Geometry: see drawing. Coordinates: mm, zero at the bounding-box minimum. A direction names the side the tool comes from. Coordinates: 2 decimals unless noted, no trailing zeros. Order: outer loops, then holes, each group sorted by start corner. A loop starts at its lowest first (then second) coordinate and runs counter-clockwise, first axis right, second up.
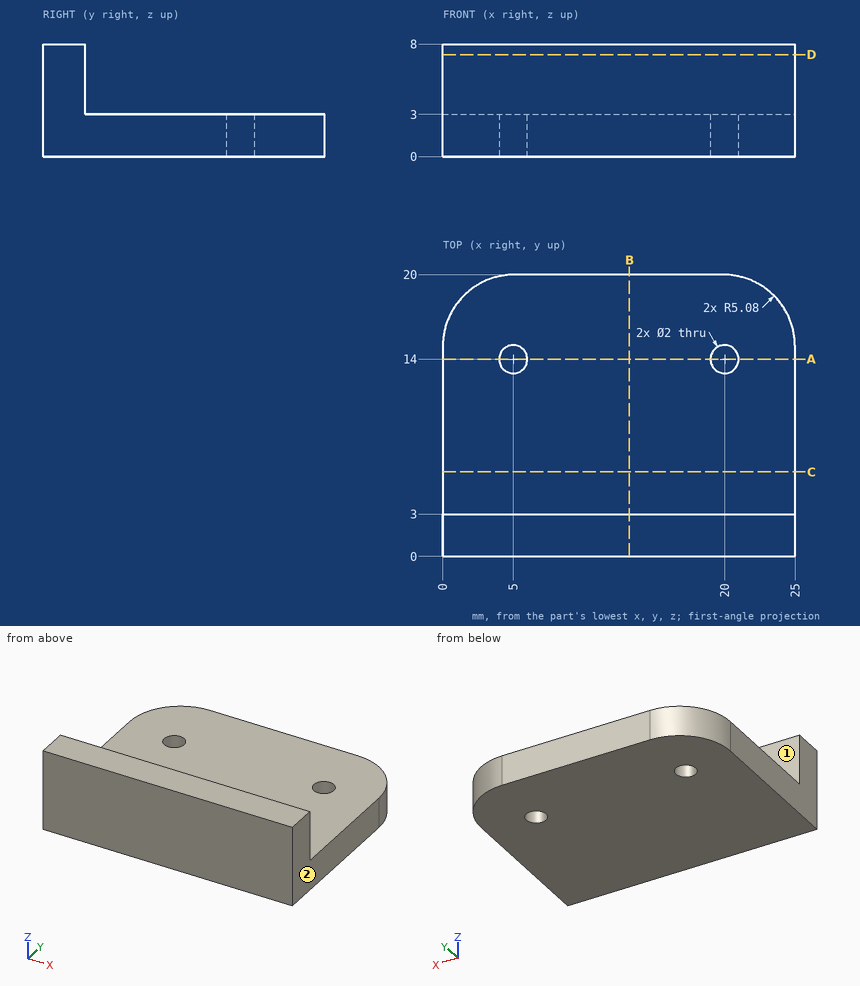
Item 1: Cut plane A-A on y = 14. Return loops of the section in (x, z).
Response values:
outline: (0, 0) - (4, 0) - (4, 3) - (0, 3) - close; (6, 0) - (19, 0) - (19, 3) - (6, 3) - close; (21, 0) - (25, 0) - (25, 3) - (21, 3) - close
Item 2: Cut plane C-C on y = 6. Return loops of the section in (x, z), then the cut area to 3 significant figures.
Response values:
outline: (0, 0) - (25, 0) - (25, 3) - (0, 3) - close
area: 75.0 mm2
Item 3: Pin query (flat end, axial travel): pin 1 Ø2.5 at (x, y) = (5, 14) entering from +Z; pin 2 Ø4 at (x, z) = (15, 6) entering from +Y. Return the tip coordinate at first contact, or that it passes through.
Response values:
pin 1: stops at z = 3
pin 2: stops at y = 3
Item 4: Access query for the marked faces 1 and 2. Directions: +Z, -Z, +X, -X, +Y, -Y. A direction counts if a zero-diameter tool reaches every point of the face in a straight line with its end or side. Return the directions, or none.
Response values:
face 1: +Z, +X, -X, +Y
face 2: +Z, -Z, +X, +Y, -Y
Item 5: Cut plane B-B on x = 13.25. Return loops of the section in (y, z), then the cut area to 3 significant figures.
Response values:
outline: (0, 0) - (20, 0) - (20, 3) - (3, 3) - (3, 8) - (0, 8) - close
area: 75.0 mm2
Item 6: Ray query, probe 1 along Y at (x, z) = (20, 0.7); probe 2 along Z at (x, y) = (12, 6.25). Return the intervals inside material, ascending.
Response values:
probe 1: y = 0 to 13, 15 to 20
probe 2: z = 0 to 3
